For this review, use the dimensioned drawing (mm, ordinates from the lowest corner) and the shaded views. Give positions to 0.01 mm unless a question says otherwise; leave off trailing zeros. Write each loop counter-clockwise with the first axis right and the second up, starting at its lowest first coordinate (ties: lowest second). Pieces come first, ordered by that corner, then holes.
1) We need section B-B on z = 20.5. Give the boundary of the cut face in (x, y).
2) We need section D-D on x = 50. Give the boundary of the cut face in (y, z).
3) Wall thickness on line 1 along X through (y, z) = (17, 12); line 2 along X through (y, z) = (23.5, 44); line 3 along X through (y, z) = (23.25, 27): over which ranges is each line inside the solid? List them lowest first.
4) Draft analysis for pull direction X (two halves, no side actions). For the marked faces 1, 2, 3 and 4, state which applies: pulls with the +X half, pulls with the -X half, needs draft (parallel to the pull), parting line crosses it, or undercut.
5) We need section C-C on z = 46. Give the boundary of the cut face in (x, y).
6) We need section A-A on y = 17.5. Give the boundary of the cut face in (x, z).
7) For P1, Ø4, axis at x = 41.5, y = 17.5, coming from the +Z side; P2, Ø10, axis at y = 8.5, z = 51, coming from the +X side; P3, Ø12.5, axis at x = 52.5, y = 14, coming from the -Z side; P4, Ø12, axis at x = 34.5, z = 64, coming from the -Y side, all flat-tipped, find the tip position at first contact; note any pin that passes through.
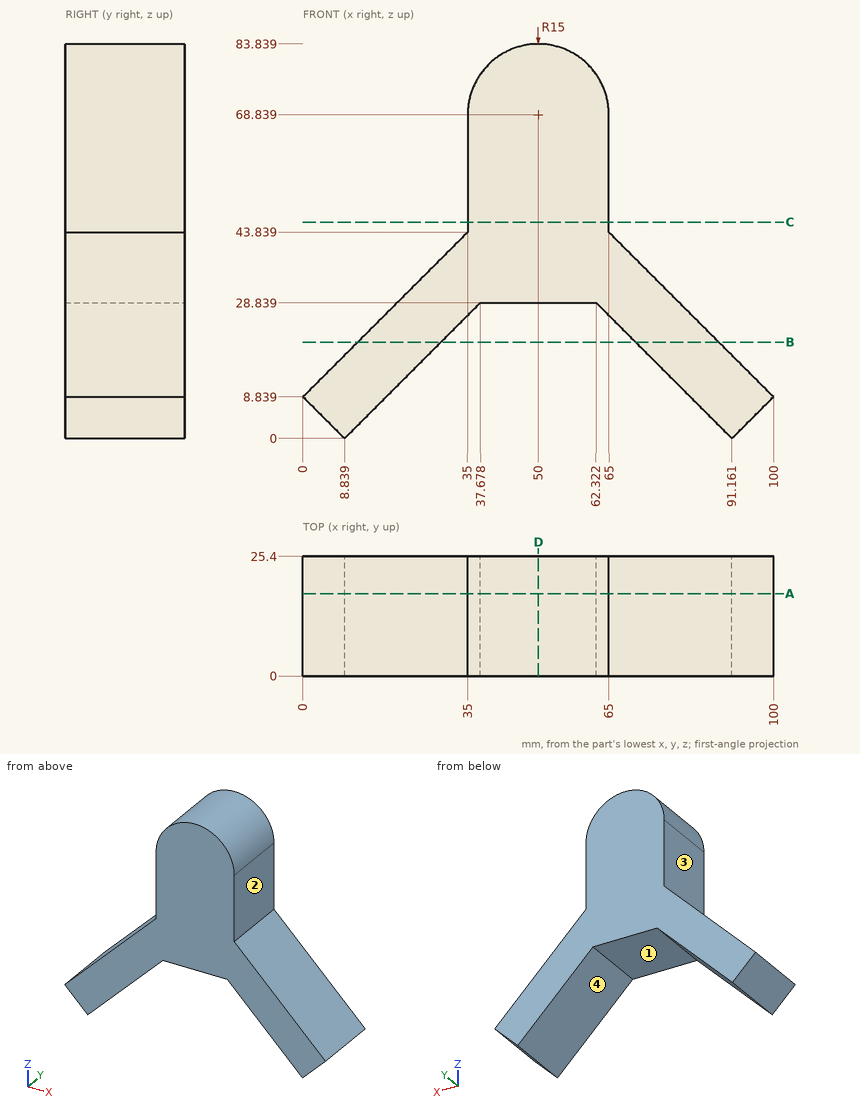
Results list:
1. outline: (11.66, 0) - (29.34, 0) - (29.34, 25.4) - (11.66, 25.4) - close; (70.66, 0) - (88.34, 0) - (88.34, 25.4) - (70.66, 25.4) - close
2. outline: (0, 28.84) - (25.4, 28.84) - (25.4, 83.84) - (0, 83.84) - close
3. line 1: x = 3.16 to 20.84, 79.16 to 96.84
3. line 2: x = 35 to 65
3. line 3: x = 18.16 to 35.84, 64.16 to 81.84
4. face 1: undercut
4. face 2: pulls with the +X half
4. face 3: pulls with the -X half
4. face 4: undercut
5. outline: (35, 0) - (65, 0) - (65, 25.4) - (35, 25.4) - close
6. outline: (0, 8.84) - (8.84, 0) - (37.68, 28.84) - (62.32, 28.84) - (91.16, 0) - (100, 8.84) - (65, 43.84) - (65, 68.84) arc R15 ccw to (35, 68.84) - (35, 43.84) - close
7. P1: stops at z = 82.36
7. P2: stops at x = 65
7. P3: stops at z = 28.84
7. P4: stops at y = 0
